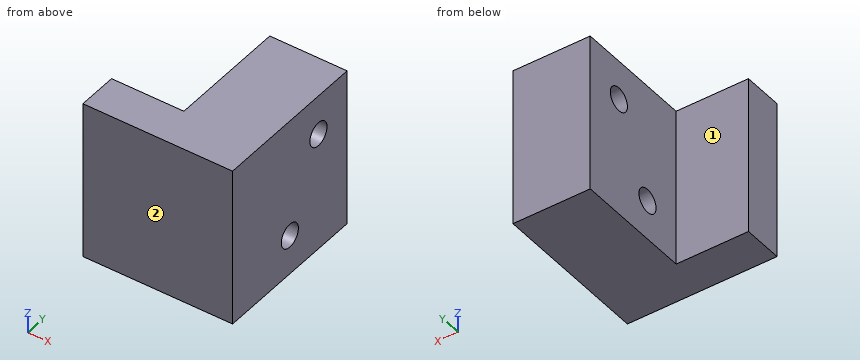
from build123d import *

# Parameters (mm, degrees)
SKETCH1_W              = 25.4
SKETCH1_H              = 25.4
EXTRUDE1_DEPTH         = 23.8125
SKETCH2_W              = 11.509375
SKETCH2_H              = 19.05
EXTRUDE2_DEPTH         = 38.060560658
F_10_24_TAPPED_HOLE1_D = 3.7973


with BuildPart() as part:
    # Sketch1 → Extrude1 (new body)
    with BuildSketch(Plane(origin=(0, 0, 0), x_dir=(0, 0, -1), z_dir=(1, 0, 0))):
        Rectangle(SKETCH1_W, SKETCH1_H)
    extrude(amount=-EXTRUDE1_DEPTH)

    # Sketch2 → Extrude2 (cut, through all)
    with BuildSketch(Plane.XY.offset(12.7)):
        with Locations((-18.0578125, 3.175)):
            Rectangle(SKETCH2_W, SKETCH2_H)
    extrude(amount=-EXTRUDE2_DEPTH, mode=Mode.SUBTRACT)

    # #10-24 Tapped Hole1 (through all)
    with Locations(Plane(origin=(-23.8125, 0.158049728, -0.576860853), x_dir=(0, 0, -1), z_dir=(-1, 0, 0))):
        with Locations((5.773139147, 0.158049728), (-6.926860853, -6.191950272)):
            Hole(F_10_24_TAPPED_HOLE1_D / 2)


solid = part.part
Input: part model. Units: mm. Frame: model coordinates. Face numbers are marked on the shaded views. A direction names the side the tool comes from. Coordinates: 2 decimals unless noted, no trailing zeros. Loops run counter-clockwise (first coordinate to the right, second up) from the corner with the lowest first, then second, coordinate; pieces in that order, holes last. Notation, with made-up numbers: (-24.75, -39.5) -> (11.25, -39.5) arc R10 ccw to (11.25, -25.5) -> close; hole circle Ø10 at (-9.75, -24.5). An arc over 180 degrees is marked (long way). Write item = value, one per line. Start each with the question number.
Item 1: Material intervals for line 1 (Y direction, x = -8.25, z = -6.35); line 2 (Y direction, x = -5.75, z = 6.35); line 3 (X direction, y = 7.25, z = 11.5), sorted ascending.
Item 2: Cut plane B-B, the plane y = 0. Return loops of the section in (x, z), plus the area to 3 significant figures.
Item 3: Reachability of the marked faces 1 and 2 from +Z, -Z, +X, -X, +Y, -Y: full face, straight path, thin tool, end or side. Return the list, or none.
Item 4: First-contact query: P1, Ø3, axis at y = 6.35, z = 6.35, coming from the -X side; P2, Ø6, axis at x = -17.5, z = -1.5, coming from the +Y side; P3, Ø4, axis at y = -1.5, z = 3, coming from the -X side. Flat tips, straight axial feed; report the tip coordinate or a pass-through.
Item 5: Cut plane C-C, the plane x = -3.75. Return loops of the section in (y, z).
Item 6: Cut plane A-A, the plane z = 6.35. Return loops of the section in (x, y).
Item 7: Cut plane D-D, the plane z = 0.25. Return loops of the section in (x, y), plus the area to 3 significant figures.
Ans:
q1.line_1 = -12.7 to -1.9, 1.9 to 12.7
q1.line_2 = -12.7 to 4.45, 8.25 to 12.7
q1.line_3 = -12.3 to 0
q2.outline = (-12.3, -12.7) -> (0, -12.7) -> (0, -8.25) -> (-12.3, -8.25) -> close; (-12.3, -4.45) -> (0, -4.45) -> (0, 12.7) -> (-12.3, 12.7) -> close
q2.area = 266 mm²
q3.face_1 = +Z, -Z, -X, +Y
q3.face_2 = +Z, -Z, +X, -X, -Y
q4.P1 = through
q4.P2 = -6.35
q4.P3 = -12.3
q5.outline = (-12.7, -12.7) -> (12.7, -12.7) -> (12.7, 12.7) -> (-12.7, 12.7) -> close; hole circle Ø3.8 at (0, -6.35); hole circle Ø3.8 at (6.35, 6.35)
q6.outline = (-23.81, -12.7) -> (0, -12.7) -> (0, 4.45) -> (-12.3, 4.45) -> (-12.3, -6.35) -> (-23.81, -6.35) -> close; (-12.3, 8.25) -> (0, 8.25) -> (0, 12.7) -> (-12.3, 12.7) -> close
q7.outline = (-23.81, -12.7) -> (0, -12.7) -> (0, 12.7) -> (-12.3, 12.7) -> (-12.3, -6.35) -> (-23.81, -6.35) -> close
q7.area = 386 mm²
